from build123d import *

# Parameters (mm, degrees)
SKETCH1_W           = 120
SKETCH1_H           = 95
BOSS_EXTRUDE1_DEPTH = 10
FILLET1_R           = 10
SKETCH3_R           = 5
BOSS_EXTRUDE3_DEPTH = 15.4
SKETCH4_W           = 15
SKETCH4_H           = 20
BOSS_EXTRUDE4_DEPTH = 16
SKETCH5_W           = 35
SKETCH5_H           = 10
BOSS_EXTRUDE5_DEPTH = 15
SKETCH6_W           = 12
SKETCH6_H           = 4
CUT_EXTRUDE1_DEPTH  = 11
SKETCH8_R           = 5.4
CUT_EXTRUDE3_DEPTH  = 11
SKETCH9_R           = 2.5
CUT_EXTRUDE4_DEPTH  = 11
CUT_EXTRUDE5_REACH  = 132
SKETCH10_R          = 4
SKETCH11_R          = 3.25
SKETCH11_R_2        = 3
CUT_EXTRUDE6_DEPTH  = 11
SKETCH12_R          = 2.5
SKETCH12_R_2        = 2.65
CUT_EXTRUDE7_DEPTH  = 5


with BuildPart() as part:
    # Sketch1 → Boss-Extrude1 (new body)
    with BuildSketch(Plane(origin=(0, 0, 0), x_dir=(1, 0, 0), z_dir=(0, 1, 0))):
        with Locations((60, 47.5)):
            Rectangle(SKETCH1_W, SKETCH1_H)
    extrude(amount=BOSS_EXTRUDE1_DEPTH)

    # Fillet1
    fillet1_edges = [part.edges().sort_by_distance(p)[0] for p in [
        (0, 5, -95),
        (120, 5, -95),
        (120, 5, 0),
        (0, 5, 0),
    ]]
    fillet(fillet1_edges, radius=FILLET1_R)

    # Sketch3 → Boss-Extrude3 (add)
    with BuildSketch(Plane(origin=(0, 10, 0), x_dir=(1, 0, 0), z_dir=(0, 1, 0))):
        with Locations((52.2, 47.5)):
            Circle(SKETCH3_R)
    extrude(amount=BOSS_EXTRUDE3_DEPTH)

    # Sketch4 → Boss-Extrude4 (add)
    with BuildSketch(Plane(origin=(0, 10, 0), x_dir=(1, 0, 0), z_dir=(0, 1, 0))):
        with Locations((107.5, 35)):
            Rectangle(SKETCH4_W, SKETCH4_H)
    extrude(amount=BOSS_EXTRUDE4_DEPTH)

    # Sketch5 → Boss-Extrude5 (add)
    with BuildSketch(Plane.ZY):
        with Locations((-47.5, 5)):
            Rectangle(SKETCH5_W, SKETCH5_H)
    extrude(amount=BOSS_EXTRUDE5_DEPTH)

    # Sketch6 → Cut-Extrude1 (cut, through all)
    with BuildSketch(Plane(origin=(0, 10, 0), x_dir=(1, 0, 0), z_dir=(0, 1, 0))):
        with Locations((-9, 47.5)):
            Rectangle(SKETCH6_W, SKETCH6_H)
    extrude(amount=-CUT_EXTRUDE1_DEPTH, mode=Mode.SUBTRACT)

    # Sketch8 → Cut-Extrude3 (cut, through all)
    with BuildSketch(Plane(origin=(0, 10, 0), x_dir=(1, 0, 0), z_dir=(0, 1, 0))):
        with Locations((7, 40)):
            Circle(SKETCH8_R)
    extrude(amount=-CUT_EXTRUDE3_DEPTH, mode=Mode.SUBTRACT)

    # Sketch9 → Cut-Extrude4 (cut, through all)
    with BuildSketch(Plane(origin=(0, 10, 0), x_dir=(1, 0, 0), z_dir=(0, 1, 0))):
        with Locations((95, 65)):
            Circle(SKETCH9_R)
    extrude(amount=-CUT_EXTRUDE4_DEPTH, mode=Mode.SUBTRACT)

    # Sketch10 → Cut-Extrude5 (cut, up to next)
    with BuildSketch(Plane(origin=(115, 0, 0), x_dir=(0, 0, -1), z_dir=(1, 0, 0)), mode=Mode.PRIVATE) as cut_extrude5_sk1:
        with Locations((35.000693392, 20.654678352)):
            Circle(SKETCH10_R)
    cut_extrude5_tool1 = extrude(cut_extrude5_sk1.sketch, amount=-CUT_EXTRUDE5_REACH, mode=Mode.PRIVATE) & part.part
    add(cut_extrude5_tool1.solids().sort_by_distance((115, 20.654678, -35.000693))[0], mode=Mode.SUBTRACT)

    # Sketch11 → Cut-Extrude6 (cut, through all)
    with BuildSketch(Plane(origin=(0, 10, 0), x_dir=(1, 0, 0), z_dir=(0, 1, 0))):
        with Locations((8, 87)):
            Circle(SKETCH11_R)
        with Locations((112, 87)):
            Circle(SKETCH11_R_2)
        with Locations((8, 8)):
            Circle(SKETCH11_R_2)
        with Locations((112, 8)):
            Circle(SKETCH11_R_2)
    extrude(amount=-CUT_EXTRUDE6_DEPTH, mode=Mode.SUBTRACT)

    # Sketch12 → Cut-Extrude7 (cut)
    with BuildSketch(Plane.XZ):
        with Locations((54.463993766, -37.5)):
            Circle(SKETCH12_R)
        with Locations((54.463993766, -57.5)):
            Circle(SKETCH12_R_2)
    extrude(amount=-CUT_EXTRUDE7_DEPTH, mode=Mode.SUBTRACT)


solid = part.part
The listing builds one solid part. Answer for the finished solid, in the listing's coordinates (mm). A direction names the side the tool comes from. Give positions to 0.01 mm unless a question says otherwise; leave off trailing zeros. Write each loop counter-clockwise with the first axis right and the second up, starting at its lowest first coordinate (ties: lowest second). Pieces come first, ordered by that corner, then holes.
1) Section C-C (y = 14.25) is taken. Write down the section's boundary in (x, z).
2) Section B-B (x = 95) is taken. Write down the section's boundary in (y, z), and give its area (3 significant figures).
3) Given P1, Ø3.5, axis at x = 8, z = -8, coming from the +Y side; P2, Ø4, axis at x = 54, z = -37.5, coming from the -Y side; P3, Ø7.5, axis at x = 109, y = 17.5, coming from the -Z side; P4, Ø8, axis at y = 3, z = -15, coming from the -X side, each flat-ended and moving along its own axis, determine where each tip first touches the part or whether it passes through.
4) Find the intervals of material crossed by L1, parallel to X at y = 6.5, z = -8; L2, parallel to Z at x = 8, y = 2.5; L3, parallel to Z at x = 7, y = 2.5, in increasing order.
5) Section A-A (y = 3.5) is taken. Count the separate pieces of the cut face and the enclosed holes in it, and give its area (3 significant figures).
6) A tool of negligible diameter and unlimited length cuts with its end or side. For faces 1 (the face through (52, 25.4, -48)), 2 (the face through (54, 5, -57)), 3 (the face through (-9, 5, -45.5)), 4 (the face through (54.888, 17.592, -51.716)), 5 (the face through (0, 5, -20)), from which of +Z, -Z, +X, -X, +Y, -Y can it reach the whole face along a straight path? Write none if from no direction.
7) Section D-D (z = -57.5) is taken. Write down the section's boundary in (x, y).
8) For a pull along X with two mould halves and no side action, classify faces 6 (the face through (107, 18, -25)), 7 (the face through (115, 16, -35)), 8 (the face through (51.817, 2.465, -57.383)) as pulls with the +X half, pulls with the -X half, needs draft (parallel to the pull), parting line crosses it, or undercut.
Response:
1. outline: circle Ø10 at (52.2, -47.5); (100, -45) - (115, -45) - (115, -25) - (100, -25) - close
2. outline: (0, -95) - (10, -95) - (10, -67.5) - (0, -67.5) - close; (0, -62.5) - (10, -62.5) - (10, 0) - (0, 0) - close
2. area: 900 mm2
3. P1: passes through
3. P2: stops at y = 5
3. P3: stops at z = -45
3. P4: stops at x = 0
4. L1: x = 0.2 to 5, 11 to 109, 115 to 119.8
4. L2: z = -94.8 to -90.25, -83.75 to -45.31, -34.69 to -11, -5 to -0.2
4. L3: z = -94.54 to -90.09, -83.91 to -45.4, -34.6 to -10.83, -5.17 to -0.46
5. separate pieces: 1
5. enclosed holes: 8
5. area: 11,500 mm2
6. face 1: +Z, -Z, -X, +Y
6. face 2: -Y
6. face 3: -X, +Y, -Y
6. face 4: +Y
6. face 5: +Z, -X, +Y, -Y
7. outline: (-15, 0) - (51.81, 0) - (51.81, 5) - (57.11, 5) - (57.11, 0) - (120, 0) - (120, 10) - (-15, 10) - close
8. face 6: needs draft
8. face 7: pulls with the +X half
8. face 8: undercut
